```python
from build123d import *

# Parameters (mm, degrees)
F1_DEPTH = 15


with BuildPart() as f1:
    # F0 (on Front) → F1 (new body)
    with BuildSketch(Plane.XZ):
        with BuildLine():
            Line((100, -87), (100, 100))
            Line((100, 100), (0, 100))
            Line((0, 100), (0, -187))
            ThreePointArc((0, -187), (2.928932, -194.071068), (10, -197))
            Line((10, -197), (220, -197))
            ThreePointArc((220, -197), (227.071068, -199.928932), (230, -207))
            Line((230, -207), (230, -384))
            ThreePointArc((230, -384), (232.928932, -391.071068), (240, -394))
            Line((240, -394), (450, -394))
            ThreePointArc((450, -394), (457.071068, -396.928932), (460, -404))
            Line((460, -404), (460, -591))
            Line((460, -591), (550, -591))
            ThreePointArc((550, -591), (557.071068, -593.928932), (560, -601))
            Line((560, -601), (560, -689))
            Line((560, -689), (660, -689))
            Line((660, -689), (660, -601))
            ThreePointArc((660, -601), (662.928932, -593.928932), (670, -591))
            Line((670, -591), (780, -591))
            ThreePointArc((780, -591), (787.071068, -588.071068), (790, -581))
            Line((790, -581), (790, -501))
            ThreePointArc((790, -501), (787.071068, -493.928932), (780, -491))
            Line((780, -491), (570, -491))
            ThreePointArc((570, -491), (562.928932, -488.071068), (560, -481))
            Line((560, -481), (560, -304))
            ThreePointArc((560, -304), (557.071068, -296.928932), (550, -294))
            Line((550, -294), (340, -294))
            ThreePointArc((340, -294), (332.928932, -291.071068), (330, -284))
            Line((330, -284), (330, -107))
            ThreePointArc((330, -107), (327.071068, -99.928932), (320, -97))
            Line((320, -97), (110, -97))
            ThreePointArc((110, -97), (102.928932, -94.071068), (100, -87))
        make_face()
    extrude(amount=F1_DEPTH)


solid = f1.part
```
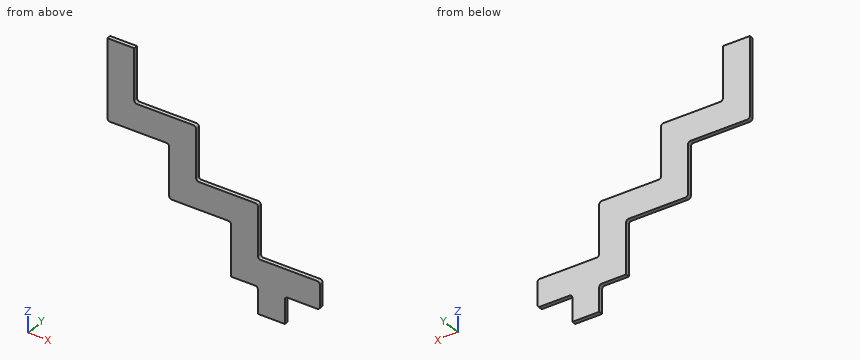
Verification items for the finished model (mm, model axes). Coordinates: 2 decimals unless noted, no trailing zeros. Loops run counter-clockwise (first coordinate to the right, second up) from the corner with the lowest first, then second, coordinate; pieces in that order, holes last. Notation, with made-up numbers: (72.5, 21.5) -> (96.5, 21.5) arc R9 cw to (96.5, 30.5) -> close; hole circle Ø1 at (4, -19.5). An arc over 180 degrees is marked (long way). Answer in a Markdown table with one row per item. Add a question column.
1. Section check C-C, the plane z = -362.5. Enter the section's corners in (x, y).
2. Section check B-B, the plane x = 63. Enter the section's corners in (y, z).
3. Material ranges on probe 1 along X at (y, z) = (-2.5, 58); probe 2 along Z at (x, y) = (680.5, -12.25); probe 3 along Z at (x, y) = (206.5, -5), recorded low to high. Write a range as [from, to].
4. Depth check by flat-ended pin: P1, Ø7.5, axis at y = -10.5, z = 49, coming from the +X side; P2, Ø7.5, axis at y = -11, z = -222.5, coming from the +X side; P3, Ø1, axis at y = -12, z = -483.5, coming from the +X side. Enter the tip coordinate at first touch or a pass-through.
Derived:
| question | item | result |
|---|---|---|
| 1 | outline | (230, -15) -> (560, -15) -> (560, 0) -> (230, 0) -> close |
| 2 | outline | (-15, -197) -> (0, -197) -> (0, 100) -> (-15, 100) -> close |
| 3 | probe 1 | x = [0, 100] |
| 3 | probe 2 | z = [-591, -491] |
| 3 | probe 3 | z = [-197, -97] |
| 4 | P1 | stops at x = 100 |
| 4 | P2 | stops at x = 330 |
| 4 | P3 | stops at x = 560.46 |
